```python
from build123d import *

# Parameters (mm, degrees)
SKETCH1_W           = 200
SKETCH1_H           = 60
BOSS_EXTRUDE1_DEPTH = 5
SKETCH2_R           = 3
CUT_EXTRUDE1_DEPTH  = 6
SKETCH3_W           = 50
SKETCH3_H           = 100
BOSS_EXTRUDE2_DEPTH = 5
CUT_EXTRUDE2_DEPTH  = 6
FILLET1_R           = 5


with BuildPart() as part:
    # Sketch1 → Boss-Extrude1 (new body)
    with BuildSketch(Plane(origin=(0, 0, 0), x_dir=(1, 0, 0), z_dir=(0, 1, 0))):
        Rectangle(SKETCH1_W, SKETCH1_H)
    extrude(amount=BOSS_EXTRUDE1_DEPTH)

    # Sketch2 → Cut-Extrude1 (cut, through all)
    with BuildSketch(Plane(origin=(0, 5, 0), x_dir=(1, 0, 0), z_dir=(0, 1, 0))):
        with Locations((-90, 20)):
            Circle(SKETCH2_R)
        with Locations((-90, -20)):
            Circle(SKETCH2_R)
        with Locations((40, -20)):
            Circle(SKETCH2_R)
        with Locations((40, 20)):
            Circle(SKETCH2_R)
        with Locations((-90, 0)):
            Circle(SKETCH2_R)
        with Locations((40, 0)):
            Circle(SKETCH2_R)
    extrude(amount=-CUT_EXTRUDE1_DEPTH, mode=Mode.SUBTRACT)

    # Sketch3 → Boss-Extrude2 (add)
    with BuildSketch(Plane(origin=(0, 0, 0), x_dir=(1, 0, 0), z_dir=(0, 1, 0))):
        with Locations((75, 0)):
            Rectangle(SKETCH3_W, SKETCH3_H)
    extrude(amount=BOSS_EXTRUDE2_DEPTH)

    # Sketch4 → Cut-Extrude2 (cut, through all)
    with BuildSketch(Plane(origin=(0, 5, 0), x_dir=(1, 0, 0), z_dir=(0, 1, 0))):
        with BuildLine():
            Line((57.5, -30.905), (92.5, -30.905))
            ThreePointArc((92.5, -30.905), (95.6, -34.005), (92.5, -37.105))
            Line((92.5, -37.105), (57.5, -37.105))
            ThreePointArc((57.5, -37.105), (54.4, -34.005), (57.5, -30.905))
        make_face()
    cut_extrude2 = extrude(amount=-CUT_EXTRUDE2_DEPTH, mode=Mode.SUBTRACT)

    # Mirror1: Cut-Extrude2 across plane
    add(cut_extrude2.mirror(Plane.XY), mode=Mode.SUBTRACT)

    # Fillet1
    fillet1_edges = [part.edges().sort_by_distance(p)[0] for p in [
        (100, 2.5, 50),
        (50, 2.5, -30),
        (50, 2.5, -50),
        (50, 2.5, 30),
        (100, 2.5, -50),
        (50, 2.5, 50),
        (-100, 2.5, 30),
        (-100, 2.5, -30),
    ]]
    fillet(fillet1_edges, radius=FILLET1_R)


solid = part.part
```
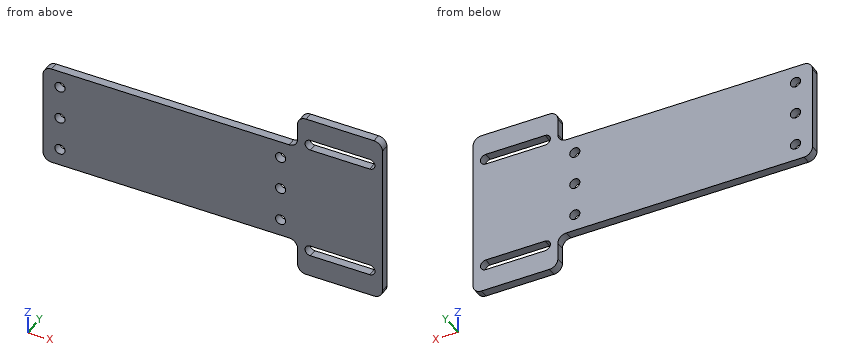
The model under review builds one solid part; all positions refer to its coordinate system, in mm. Round coordinates to 2 decimals unless told otherwise and drop trailing zeros. Write each loop counter-clockwise with the first axis right and the second up, starting at its lowest first coordinate (ties: lowest second). Pieces come first, ordered by that corner, then holes. Notation, with made-up numbers: (84, -25.75) - (102, -25.75) arc R22 cw to (102, 0.25) - close; hole circle Ø4 at (79.5, 16). An arc over 180 degrees is marked (long way). Answer as CSV lines item,"result". Start each with the question number.
(1) We need section C-C on x = 78.5. State the section outline as (y, z) points (3 decimals).
(2) We need section D-D on y = 0.8. Give the number of separate pieces and of enclosed holes in the cut face, plus the area to 3 significant figures.
(3) For pin 1 Ø5 at (x, z) = (-90, 0) entering from +Y; pin 2 Ø1.5 at (x, y) = (7, 2.5) entering from -Z; pin 3 Ø2.5 at (y, z) = (3, -40) entering from -X, all flat-tipped, find the tip position at first contact; note any pin that passes through.
(4) We need section B-B on z = 0. State the section outline as (x, y) points, plus the area to 3 significant figures.
(5) We need section A-A on x = 40. State the section outline as (y, z) points.
(6) To check wall thickness, follow line 1 (Z direction, x = -90, y = 2.3); line 2 (X direction, y = 3.75, z = 0); line 3 (Z direction, x = 64, y = 1.6) (3 decimals). State the ranges of each line that lie inside material, in increasing order.
Worked answers:
1,outline,"(0, -50) - (5, -50) - (5, -37.105) - (0, -37.105) - close; (0, -30.905) - (5, -30.905) - (5, 30.905) - (0, 30.905) - close; (0, 37.105) - (5, 37.105) - (5, 50) - (0, 50) - close"
2,separate pieces,"1"
2,enclosed holes,"8"
2,area,"13,300 mm²"
3,pin 1,"through"
3,pin 2,"z = -30"
3,pin 3,"x = 50"
4,outline,"(-100, 0) - (-93, 0) - (-93, 5) - (-100, 5) - close; (-87, 0) - (37, 0) - (37, 5) - (-87, 5) - close; (43, 0) - (100, 0) - (100, 5) - (43, 5) - close"
4,area,"940 mm²"
5,outline,"(0, -30) - (5, -30) - (5, -23) - (0, -23) - close; (0, -17) - (5, -17) - (5, -3) - (0, -3) - close; (0, 3) - (5, 3) - (5, 17) - (0, 17) - close; (0, 23) - (5, 23) - (5, 30) - (0, 30) - close"
6,line 1,"-30 to -23, -17 to -3, 3 to 17, 23 to 30"
6,line 2,"-100 to -93, -87 to 37, 43 to 100"
6,line 3,"-50 to -37.105, -30.905 to 30.905, 37.105 to 50"
